from build123d import *

# Parameters (mm, degrees)
SKETCH_1_W          = 29
SKETCH_1_H          = 18
SKETCH_1_R          = 1.7
EXTRUDE_1_DEPTH     = 4.8
SKETCH_2_W          = 0.5
SKETCH_2_H          = 1
CUT_EXTRUDE_1_DEPTH = 35.467956133


with BuildPart() as part:
    # 草图1 → 凸台-拉伸1 (new body)
    with BuildSketch(Plane.XY):
        with Locations((14.5, 9)):
            Rectangle(SKETCH_1_W, SKETCH_1_H)
        with Locations((21.5, 7)):
            Circle(SKETCH_1_R, mode=Mode.SUBTRACT)
        with Locations(Location((7.5, 7, 0), (0, 0, 180))):
            Circle(SKETCH_1_R, mode=Mode.SUBTRACT)
    extrude(amount=EXTRUDE_1_DEPTH)

    # 草图2 → 切除-拉伸1 (cut, through all)
    with BuildSketch(Plane(origin=(0, 18, 0), x_dir=(1, 0, 0), z_dir=(0, 1, 0))):
        Polygon((0, -4.8), (1, -4.8), (1, -3.8), (0.5, -3.8), (0, -3.8), align=None)
        Polygon((2, -4.8), (3, -4.8), (3, -3.8), (2.5, -3.8), (2, -3.8), align=None)
        Polygon((4, -4.8), (5, -4.8), (5, -3.8), (4.5, -3.8), (4, -3.8), align=None)
        Polygon((6, -4.8), (7, -4.8), (7, -3.8), (6.5, -3.8), (6, -3.8), align=None)
        Polygon((8, -4.8), (9, -4.8), (9, -3.8), (8.5, -3.8), (8, -3.8), align=None)
        Polygon((10, -4.8), (11, -4.8), (11, -3.8), (10.5, -3.8), (10, -3.8), align=None)
        Polygon((12, -4.8), (13, -4.8), (13, -3.8), (12.5, -3.8), (12, -3.8), align=None)
        with Locations((14.75, -4.3)):
            Rectangle(SKETCH_2_W, SKETCH_2_H)
        with Locations((14.25, -4.3)):
            Rectangle(SKETCH_2_W, SKETCH_2_H)
        Polygon((16, -3.8), (16, -4.8), (17, -4.8), (17, -3.8), (16.5, -3.8), align=None)
        Polygon((18, -3.8), (18, -4.8), (19, -4.8), (19, -3.8), (18.5, -3.8), align=None)
        Polygon((20, -3.8), (20, -4.8), (21, -4.8), (21, -3.8), (20.5, -3.8), align=None)
        Polygon((22, -3.8), (22, -4.8), (23, -4.8), (23, -3.8), (22.5, -3.8), align=None)
        Polygon((24, -3.8), (24, -4.8), (25, -4.8), (25, -3.8), (24.5, -3.8), align=None)
        Polygon((26, -3.8), (26, -4.8), (27, -4.8), (27, -3.8), (26.5, -3.8), align=None)
        Polygon((28, -3.8), (28, -4.8), (29, -4.8), (29, -3.8), (28.5, -3.8), align=None)
    extrude(amount=-CUT_EXTRUDE_1_DEPTH, mode=Mode.SUBTRACT)


solid = part.part
Read the model definition and answer for the solid it produces. Units are mm, in the model's axes. A direction names the side the tool comes from. Give positions to 0.01 mm unless a question says otherwise; leave off trailing zeros. Write each loop counter-clockwise with the first axis right and the second up, starting at its lowest first coordinate (ties: lowest second). Pieces come first, ordered by that corner, then holes. Notation, with made-up numbers: (48.5, -20.5) - (59.5, -20.5) arc R22 cw to (59.5, 8.5) - close; hole circle Ø2 at (23, 60.25). An arc over 180 degrees is marked (long way). Answer in a Markdown table with one row per item. Add a question column.
Item 1: Determine the mould class of faces 1 (the face through (14, 0, 2)), 2 (the face through (5.93, 7.65, 2.37)), 3 (the face through (23, 3, 4)) for opening direction Y: pulls with the +Y half, pulls with the -Y half, needs draft (parallel to the pull), parting line crosses it, or undercut.
Item 2: Flat-ended cylindrical pins translate along their axes: P1, Ø1.1, axis at y = 8.5, z = 4.5, coming from the -X side; P2, Ø4, axis at x = 24.5, y = 6.5, coming from the +Z side; P3, Ø0.8, axis at x = 22.5, y = 3, coming from the +Z side; P4, Ø1.1, axis at y = 12, z = 4.5, coming from the +X side. Find the tip coordinate at first contact, or state that the pin passes through.
Item 3: Section B-B, the plane z = 1.2 is taken. Write down the section's boundary in (x, y), and give its area (3 significant figures).
Item 4: Find the intervals of material crossed by L1, parallel to X at y = 7, z = 2.8; L2, parallel to Y at x = 7.5, z = 1.85; L3, parallel to Y at x = 23, z = 0.6, in increasing order.
Item 5: Section A-A, the plane x = 21.5 is taken. Write down the section's boundary in (y, z), and give its area (3 significant figures).
Item 6: A tool of negligible diameter and unlimited length cuts with its end or side. For faces 4 (the face through (7.5, 13.4, 4.8)), 5 (the face through (8, 13, 4)), from which of +Z, -Z, +X, -X, +Y, -Y can it reach the whole face along a straight path? Write none if from no direction.
Item 7: Section C-C, the plane y = 7 is taken. Count the separate pieces of the cut face and the enclosed holes in it, and give its area (3 significant figures).
Recorded:
| question | item | result |
|---|---|---|
| 1 | face 1 | pulls with the -Y half |
| 1 | face 2 | undercut |
| 1 | face 3 | needs draft |
| 2 | P1 | stops at x = 1 |
| 2 | P2 | stops at z = 4.8 |
| 2 | P3 | stops at z = 3.8 |
| 2 | P4 | stops at x = 28 |
| 3 | outline | (0, 0) - (29, 0) - (29, 18) - (0, 18) - close; hole circle Ø3.4 at (7.5, 7); hole circle Ø3.4 at (21.5, 7) |
| 3 | area | 504 mm2 |
| 4 | L1 | x = 0 to 5.8, 9.2 to 19.8, 23.2 to 29 |
| 4 | L2 | y = 0 to 5.3, 8.7 to 18 |
| 4 | L3 | y = 0 to 6.2, 7.8 to 18 |
| 5 | outline | (0, 0) - (5.3, 0) - (5.3, 4.8) - (0, 4.8) - close; (8.7, 0) - (18, 0) - (18, 4.8) - (8.7, 4.8) - close |
| 5 | area | 70.1 mm2 |
| 6 | face 4 | +Z, +X, -X, +Y, -Y |
| 6 | face 5 | +Z, +Y, -Y |
| 7 | separate pieces | 3 |
| 7 | enclosed holes | 0 |
| 7 | area | 95.6 mm2 |
